Work out the finished part from the listing and answer in its coordinate system (mm). Round coordinates to 2 decimals unless told otherwise and drop trailing zeros. Loops run counter-clockwise (first coordinate to the right, second up) from the corner with the lowest first, then second, coordinate; pieces in that order, holes last.
```python
from build123d import *

# Parameters (mm, degrees)
BOSS_EXTRUDE1_DEPTH = 12.7
SKETCH2_R           = 6.35
CUT_EXTRUDE1_DEPTH  = 182.323455578


with BuildPart() as part:
    # Sketch1 → Boss-Extrude1 (new body)
    with BuildSketch(Plane(origin=(0, 0, 0), x_dir=(1, 0, 0), z_dir=(0, 1, 0))):
        with BuildLine():
            Line((-131.471489953, 109.23134636), (71.728510047, 109.23134636))
            ThreePointArc((71.728510047, 109.23134636), (80.708766168, 105.511602481), (84.428510047, 96.53134636))
            Line((84.428510047, 96.53134636), (84.428510047, 38.349564826))
            ThreePointArc((84.428510047, 38.349564826), (83.442873319, 33.444088994), (80.638952072, 29.300033185))
            Line((80.638952072, 29.300033185), (10.746499625, -39.518185281))
            ThreePointArc((10.746499625, -39.518185281), (6.650668081, -42.220654573), (1.836057601, -43.16865364))
            Line((1.836057601, -43.16865364), (-63.841823784, -43.16865364))
            ThreePointArc((-63.841823784, -43.16865364), (-68.748013198, -42.182718068), (-72.892440933, -39.377993078))
            Line((-72.892440933, -39.377993078), (-140.522107103, 29.324094297))
            ThreePointArc((-140.522107103, 29.324094297), (-143.22378415, 33.419539146), (-144.171489953, 38.233433734))
            Line((-144.171489953, 38.233433734), (-144.171489953, 96.53134636))
            ThreePointArc((-144.171489953, 96.53134636), (-140.451746074, 105.511602481), (-131.471489953, 109.23134636))
        make_face()
    extrude(amount=BOSS_EXTRUDE1_DEPTH)

    # Sketch2 → Cut-Extrude1 (cut, through all)
    with BuildSketch(Plane(origin=(0, 12.7, 0), x_dir=(1, 0, 0), z_dir=(0, 1, 0))):
        with Locations(Location((-69.102883091, -30.46865364, 0), (0, 0, 270))):
            Circle(SKETCH2_R)
        with Locations(Location((7.097116909, -30.46865364, 0), (0, 0, 270))):
            Circle(SKETCH2_R)
        with Locations(Location((-67.971489953, 96.53134636, 0), (0, 0, 270))):
            Circle(SKETCH2_R)
        with Locations(Location((8.228510047, 96.53134636, 0), (0, 0, 270))):
            Circle(SKETCH2_R)
        with Locations(Location((-67.971489286, 33.021266411, 0), (0, 0, 270))):
            Circle(SKETCH2_R)
        with Locations(Location((8.228510047, 33.03134636, 0), (0, 0, 270))):
            Circle(SKETCH2_R)
        with Locations(Location((-131.471489953, 96.53134636, 0), (0, 0, 270))):
            Circle(SKETCH2_R)
        with Locations(Location((-131.471489953, 33.03134636, 0), (0, 0, 270))):
            Circle(SKETCH2_R)
        with Locations(Location((71.728510047, 96.53134636, 0), (0, 0, 270))):
            Circle(SKETCH2_R)
        with Locations(Location((71.728510047, 33.03134636, 0), (0, 0, 270))):
            Circle(SKETCH2_R)
        with Locations(Location((-29.871490619, 33.03134636, 0), (0, 0, 270))):
            Circle(SKETCH2_R)
    extrude(amount=-CUT_EXTRUDE1_DEPTH, mode=Mode.SUBTRACT)


solid = part.part
```
1. Consider probe 1 along X at (y, z) = (4, -31.5); probe 2 along Z at (x, y) = (-72.5, 10.5); probe 3 along X at (y, z) = (9, -35). Determine where each line is inside the solid, lowest interval first.
Answer key:
probe 1: x = -142.24 to -137.63, -125.31 to -74.14, -61.81 to -36.03, -23.71 to 2.07, 14.39 to 65.57, 77.89 to 82.42
probe 2: z = -109.23 to -100.98, -92.08 to -37.47, -28.57 to 25.1, 35.83 to 39.76
probe 3: x = -143.75 to -137.51, -125.43 to -74.01, -61.94 to -35.91, -23.83 to 2.19, 14.27 to 65.69, 77.77 to 83.98
2. Given pin 1 (7.5 mm diameter, centred on x = -131.47, z = -96.53, fed in from +Y); pin 2 (6 mm diameter, centred on y = 3.5, z = -24, fed in from +X); pin 3 (2 mm diameter, centred on y = 1.5, z = -19, fed in from -X); pin 4 (1.5 mm diameter, centred on y = 11.5, z = -35.5, fed in from -X), each flat-ended and moving along its own axis, determine where each tip first touches the part or whether it passes through.
Answer key:
pin 1: passes through
pin 2: stops at x = 78.3
pin 3: stops at x = -131.34
pin 4: stops at x = -144.02
3. Find section C-C (x = 18). Write down the section's boundary in (y, z), then the cut area to 3 significant figures.
Answer key:
outline: (0, -109.23) - (12.7, -109.23) - (12.7, 32.38) - (0, 32.38) - close
area: 1,800 mm2
4. Determine the mould class of faces 1 (the face through (73.636, 6.439, -90.475)), 2 (the face through (46.18, 6.26, 4.63)), 3 (the face through (-28, 12.7, -51)) for opening direction Z: +Z half, -Z half, draft (parallel to the pull), parting line (faces both ways), or undercut.
Answer key:
face 1: undercut
face 2: +Z half
face 3: draft
5. Find section A-A (z = 34.5). Write down the section's boundary in (x, y).
Answer key:
outline: (-77.69, 0) - (-74.01, 0) - (-74.01, 12.7) - (-77.69, 12.7) - close; (-64.2, 0) - (2.19, 0) - (2.19, 12.7) - (-64.2, 12.7) - close; (12, 0) - (15.84, 0) - (15.84, 12.7) - (12, 12.7) - close
6. Find section D-D (z = -23.5). Write down the section's boundary in (x, y).
Answer key:
outline: (-134.79, 0) - (74.75, 0) - (74.75, 12.7) - (-134.79, 12.7) - close
7. Find section B-B (y = 3.5). Give the number of separate pieces and of enclosed holes in the cut face, then the cut area to 3 significant figures.
Answer key:
separate pieces: 1
enclosed holes: 11
area: 27,600 mm2
